Solid Edge part; units mm, degrees
sketch "Sketch1" plane through (0, 0, 0) normal (0, -1, 0) x (1, 0, 0)
  line L0 (-6.5, -5.5) -> (6.5, -5.5)
  line L1 (6.5, -5.5) -> (6.5, 5.5)
  line L2 (6.5, 5.5) -> (-6.5, 5.5)
  line L3 (-6.5, 5.5) -> (-6.5, -5.5)
  dimension "D1" = 6.5
  dimension "D2" = 6.5
extrude "Protrusion1" add sketch "Sketch1" against normal blind 1.5
sketch "Sketch2" plane through (0, 0, 0) normal (0, -1, 0) x (1, 0, 0)
  line L0 (-6.5, 5.5) -> (6.5, 5.5)
  line L1 (6.5, 5.5) -> (6.5, 3.5)
  line L2 (6.5, 3.5) -> (-6.5, 3.5)
  line L3 (-6.5, 3.5) -> (-6.5, 5.5)
  line L4 (-6.5, -5.5) -> (6.5, -5.5)
  line L5 (6.5, -5.5) -> (6.5, -3.5)
  line L6 (6.5, -3.5) -> (-6.5, -3.5)
  line L7 (-6.5, -3.5) -> (-6.5, -5.5)
  dimension "D1" = 6.5
  dimension "D2" = 6.5
extrude "side" add sketch "Sketch2" along normal blind 7
sketch "Sketch3" plane through (0, -2.75, 5.5) normal (0, 0, 1) x (-1, 0, 0)
  line L0 (-6.5, 4.25) -> (-1.5, 4.25)
  line L1 (-1.5, 4.25) -> (-1.5, -4.25)
  line L2 (-1.5, -4.25) -> (-6.5, -4.25)
  line L3 (-6.5, -4.25) -> (-6.5, 4.25)
  dimension "D1" = 6.5
extrude "Extrusionsausschnitt_1" cut sketch "Sketch3" against normal blind 2
sketch "Sketch4" plane through (0, 0, 0) normal (0, -1, 0) x (-1, 0, 0)
  line L0 (-1.5, -3.5) -> (-6.5, 0)
  line L1 (-6.5, 0) -> (-6.5, -3.5)
  line L2 (-6.5, -3.5) -> (-1.5, -3.5)
extrude "Cutout1" cut sketch "Sketch4" against normal up to next
sketch "Sketch5" plane through (0, -7, -4.5) normal (0, -1, 0) x (-1, 0, 0)
  line L0 (-6.5, 1) -> (-6, 1)
  line L1 (-6, 1) -> (-6, -1)
  line L2 (-6, -1) -> (-6.5, -1)
  line L3 (-6.5, -1) -> (-6.5, 1)
  line L4 (6.5, 1) -> (6, 1)
  line L5 (6, 1) -> (6, -1)
  line L6 (6, -1) -> (6.5, -1)
  line L7 (6.5, -1) -> (6.5, 1)
  line L8 (6.5, -8) -> (6, -8)
  line L9 (6, -8) -> (6, -10)
  line L10 (6, -10) -> (6.5, -10)
  line L11 (6.5, -10) -> (6.5, -8)
  line L12 (-1.5, -8) -> (-1, -8)
  line L13 (-1, -8) -> (-1, -10)
  line L14 (-1, -10) -> (-1.5, -10)
  line L15 (-1.5, -10) -> (-1.5, -8)
  dimension "D1" = 6.5
extrude "Cutout2" cut sketch "Sketch5" against normal up to vertex (7 mm away)
chamfer "Fase_1" distance 1 angle 45 2 edges at (0, -7, -3.5) (-2.5, -7, 3.5)
properties material "Nylon, allgemein"
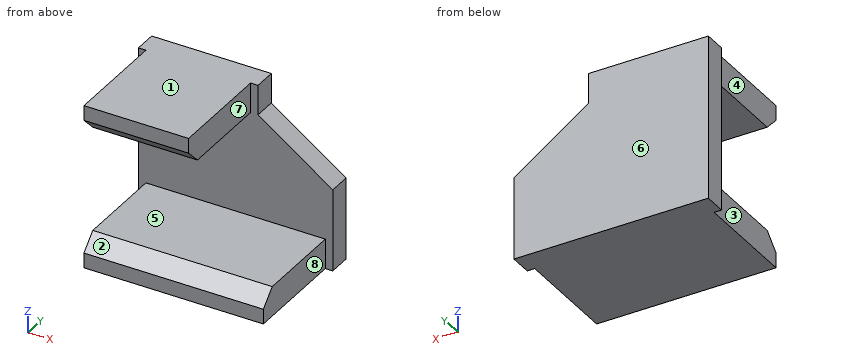
Input: part model. Units: mm. Frame: model coordinates. Face numbers are marked on the shaded views. A direction names the side the tool comes from. Give positions to 0.01 mm unless a question says otherwise; leave off trailing zeros. Order: outer loops, then holes, each group sorted by start corner. A loop starts at its lowest first (then second) coordinate and runs counter-clockwise, first axis right, second up.
1. Set-up query: the marked faces 4, 5, 6, 7 and 8. Return all of +Z, -Z, +X, -X, +Y, -Y with unobstructed straight access to the full face (end or side cutting, diameter ignored); none if empty.
Computed:
face 4: +Z, -Z, -X, -Y
face 5: +X, -X, -Y
face 6: +Z, -Z, +X, -X, +Y
face 7: +Z, +X, -Y
face 8: +Z, -Z, +X, -Y
2. Line query: probe 1 along Z at (x, y) = (-4, -0.5); probe 2 along Y at (x, z) = (6, -2.5); probe 3 along Y at (x, z) = (-5.5, -4). Output: solid intervals per line, ascending.
Computed:
probe 1: z = -5.5 to -3.5, 3.5 to 5.5
probe 2: y = 0 to 1.5
probe 3: y = -6.5 to 1.5
3. Pin query (flat end, axial travel): pin 1 Ø2 at (x, z) = (-4, -0.5) entering from -Y; pin 2 Ø2 at (y, z) = (-2, -5) entering from -X; pin 3 Ø1.6 at (y, z) = (-4, -4) entering from +X. Return the tip coordinate at first contact, or that it passes through.
Computed:
pin 1: stops at y = 0
pin 2: stops at x = -6
pin 3: stops at x = 6
4. Cut plane D-D (y = 0.5). Return loops of the section in (x, z), and give its area (3 significant figures).
Computed:
outline: (-6.5, -5.5) - (6.5, -5.5) - (6.5, 0) - (1.5, 3.5) - (1.5, 5.5) - (-6.5, 5.5) - close
area: 124 mm2
5. Cut plane C-C (z = 4.25). Return loops of the section in (x, y).
Computed:
outline: (-6.5, 0) - (-6, 0) - (-6, -6.75) - (1, -6.75) - (1, 0) - (1.5, 0) - (1.5, 1.5) - (-6.5, 1.5) - close
6. Draft query along Z for the marked faces 1, 2 and 3. Return one class per face: released by +Z, released by -Z, zero draft, split by the parting line, or undercut.
Computed:
face 1: released by +Z
face 2: undercut
face 3: zero draft
7. Cut plane A-A (y = -5). Return loops of the section in (x, z).
Computed:
outline: (-6, -5.5) - (6, -5.5) - (6, -3.5) - (-6, -3.5) - close; (-6, 3.5) - (1, 3.5) - (1, 5.5) - (-6, 5.5) - close
8. Cut plane B-B (x = -1.25). Return loops of the section in (y, z), and give its area (3 significant figures).
Computed:
outline: (-7, -5.5) - (1.5, -5.5) - (1.5, 5.5) - (-7, 5.5) - (-7, 4.5) - (-6, 3.5) - (0, 3.5) - (0, -3.5) - (-6, -3.5) - (-7, -4.5) - close
area: 43.5 mm2
